```python
from build123d import *

# Parameters (mm, degrees)
SKETCH2_R           = 10
BOSS_EXTRUDE1_DEPTH = 15
SKETCH3_R           = 7.5
BOSS_EXTRUDE2_DEPTH = 10
SKETCH8_R           = 7.5
BOSS_EXTRUDE3_DEPTH = 30
SKETCH4_W           = 35
SKETCH4_H           = 315
SKETCH9_W           = 70
SKETCH9_H           = 80
CUT_EXTRUDE1_DEPTH  = 15


with BuildPart() as part:
    # Sketch1 → Base-Revolve (revolve)
    with BuildSketch(Plane.XY):
        Polygon((22.5, -330), (40, -330), (40, -10), (45, -10), (45, 40), (50, 40), (50, 70), (0, 70), (0, 55), (35, 55), (35, -325), (22.5, -325), align=None)
    revolve(axis=Axis((0, 100, 0), (0, -1, 0)))

    # Sketch2 → Boss-Extrude1 (add, symmetric)
    with BuildSketch(Plane.XY):
        with BuildLine():
            Line((19.138857956, 105.805524623), (30, 70))
            Line((30, 70), (-30, 70))
            Line((-30, 70), (-19.138857956, 105.805524623))
            ThreePointArc((-19.138857956, 105.805524623), (0, 120), (19.138857956, 105.805524623))
        make_face()
        with Locations((0, 100)):
            Circle(SKETCH2_R, mode=Mode.SUBTRACT)
    extrude(amount=BOSS_EXTRUDE1_DEPTH, both=True)

    # Sketch3 → Boss-Extrude2 (add, symmetric)
    with BuildSketch(Plane.XY):
        with BuildLine():
            Line((62.373967528, -280.189048708), (30, -275))
            Line((30, -275), (30, -315))
            Line((30, -315), (62.373967528, -309.810951292))
            ThreePointArc((62.373967528, -309.810951292), (75, -295), (62.373967528, -280.189048708))
        make_face()
        with Locations((60, -295)):
            Circle(SKETCH3_R, mode=Mode.SUBTRACT)
    boss_extrude2 = extrude(amount=BOSS_EXTRUDE2_DEPTH, both=True)

    # Mirror1: Boss-Extrude2 across plane
    add(boss_extrude2.mirror(Plane(origin=(0, 0, 0), x_dir=(0, 0, 1), z_dir=(1, 0, 0))))

    # Sketch8 → Boss-Extrude3 (add, symmetric)
    with BuildSketch(Plane.XY):
        with BuildLine():
            Line((82.041582998, -85.08350067), (20, -80))
            Line((20, -80), (20, -140))
            Line((20, -140), (82.041582998, -134.91649933))
            ThreePointArc((82.041582998, -134.91649933), (105, -110), (82.041582998, -85.08350067))
        make_face()
        with Locations((80, -110)):
            Circle(SKETCH8_R, mode=Mode.SUBTRACT)
    extrude(amount=BOSS_EXTRUDE3_DEPTH, both=True)

    # Sketch4 → Cut-Revolve1 (revolve, cut)
    with BuildSketch(Plane.XY):
        with Locations((17.5, -167.5)):
            Rectangle(SKETCH4_W, SKETCH4_H)
    revolve(axis=Axis((0, 0, 0), (0, -1, 0)), mode=Mode.SUBTRACT)

    # Sketch9 → Cut-Extrude1 (cut, symmetric)
    with BuildSketch(Plane.XY):
        with Locations((95, -110)):
            Rectangle(SKETCH9_W, SKETCH9_H)
    extrude(amount=CUT_EXTRUDE1_DEPTH, both=True, mode=Mode.SUBTRACT)


solid = part.part
```
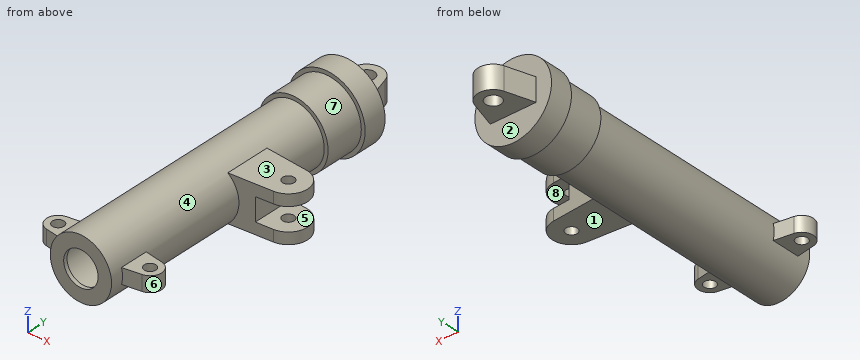
CAD build for the part. Positions are in the model's coordinates, mm. Face numbers are marked on the shaded views. A direction names the side the tool comes from. Round coordinates to 2 decimals unless told otherwise and drop trailing zeros. Order: outer loops, then holes, each group sorted by start corner. A loop starts at its lowest first (then second) coordinate and runs counter-clockwise, first axis right, second up.
Q1. Slice it at C-C (y = 0). Write the cut outline in (x, z).
Q2. Which spindle directions (+Z, -Z, +X, -X, +Y, -Y) get a long thin tool onto all of the face, cutting with end or side? Do the marked faces 1, 2, 3, 4 and 5. Say none if no direction does.
Q3. Drop flat-ended pins along their axis: pin 1 (17 mm diameter, centred on x = 80, y = -110, fed in from +Z); pin 2 (18 mm diameter, centred on x = 0, y = 100, fed in from +Z); pin 3 (24 mm diameter, centred on x = 60, y = -295, fed in from -Z); pin 4 (24 mm diameter, centred on x = 80, y = -110, fed in from -Z). Give the stop position or say it passes through.
Q4. Two-plate mould, pull along Z, no slides. Class the marked faces 6, 7 and 8: pulls with the +Z half, pulls with the -Z half, needs draft (parallel to the pull), parting line crosses it, or undercut.
Q5. Slice it at B-B (y = 100). Write the cut outline in (x, z).
Q6. Slice it at D-D (z = 0). State how many separate pieces and enclosed holes the cut face has, and give its area (3 significant figures).
Q7. Wall check: L1, parallel to X at y = -295, z = -1.25; L2, parallel to X at y = -295, z = 2.25; L3, parallel to Z at x = 0, y = -215. Give the ranges that are in metal, low to high.
Q8. Slice it at A-A (x = 0). Write the cut outline in (y, z).
Results below:
1. outline: circle Ø90 at (0, 0); hole circle Ø70 at (0, 0)
2. face 1: -Z, +X, -Y
2. face 2: +Y
2. face 3: +Z, +X, -Y
2. face 4: none
2. face 5: +X, +Y, -Y
3. pin 1: stops at z = 30
3. pin 2: passes through
3. pin 3: stops at z = -10
3. pin 4: stops at z = -30
4. face 6: needs draft
4. face 7: parting line crosses it
4. face 8: undercut
5. outline: (-20.9, -15) - (-10, -15) - (-10, 15) - (-20.9, 15) - close; (10, -15) - (20.9, -15) - (20.9, 15) - (10, 15) - close
6. separate pieces: 1
6. enclosed holes: 3
6. area: 10,900 mm2
7. L1: x = -75 to -67.5, -52.5 to -34.98, 34.98 to 52.5, 67.5 to 75
7. L2: x = -75 to -67.5, -52.5 to -34.93, 34.93 to 52.5, 67.5 to 75
7. L3: z = -40 to -35, 35 to 40
8. outline: (-330, -40) - (-10, -40) - (-10, -45) - (40, -45) - (40, -50) - (70, -50) - (70, -15) - (90, -15) - (90, 15) - (70, 15) - (70, 50) - (40, 50) - (40, 45) - (-10, 45) - (-10, 40) - (-330, 40) - (-330, 22.5) - (-325, 22.5) - (-325, 35) - (55, 35) - (55, -35) - (-325, -35) - (-325, -22.5) - (-330, -22.5) - close; (110, -15) - (120, -15) - (120, 15) - (110, 15) - close
